Read the model definition and answer for the solid it produces. Units are mm, in the model's axes. Coordinates: 2 decimals unless noted, no trailing zeros. Order: outer loops, then holes, each group sorted by start corner. A loop starts at its lowest first (then second) coordinate and runs counter-clockwise, first axis right, second up. Notation, with made-up numbers: (69, -31.5) -> (102, -31.5) arc R28 ccw to (102, -11.5) -> close; hole circle Ø6 at (-30, 26.5). An arc over 180 degrees is marked (long way). Return JSON: item names as keys, results as strings. Group by question number.
```python
from build123d import *

# Parameters (mm, degrees)
SKETCH1_R           = 2
BOSS_EXTRUDE1_DEPTH = 32.766
SKETCH2_W           = 0.5
SKETCH2_H           = 0.2
SKETCH3_W           = 0.15
SKETCH3_H           = 0.2
CUT_EXTRUDE1_DEPTH  = 3


with BuildPart() as part:
    # Sketch1 → Boss-Extrude1 (new body)
    with BuildSketch(Plane(origin=(0, 0, 0), x_dir=(1, 0, 0), z_dir=(0, 1, 0))):
        Circle(SKETCH1_R)
    extrude(amount=BOSS_EXTRUDE1_DEPTH)

    # Sketch2 → Cut-Revolve1 (revolve, cut)
    with BuildSketch(Plane(origin=(0, 0, 0), x_dir=(0, 0, -1), z_dir=(1, 0, 0))):
        with Locations((1.75, 0.9)):
            Rectangle(SKETCH2_W, SKETCH2_H)
    revolve(axis=Axis((0, 0, 0), (0, 1, 0)), mode=Mode.SUBTRACT)

    # Sketch3 → Cut-Extrude1 (cut)
    with BuildSketch(Plane(origin=(0, 32.766, 0), x_dir=(1, 0, 0), z_dir=(0, 1, 0))):
        with Locations((-1.925, 0)):
            Rectangle(SKETCH3_W, SKETCH3_H)
    extrude(amount=-CUT_EXTRUDE1_DEPTH, mode=Mode.SUBTRACT)


solid = part.part
```
1. Find section C-C on y = 17.5. Determine the outline of the cut face in (x, z), and give its area (3 significant figures).
2. Straight lines are drawn through the part: L1, parallel to Y at x = 1.4, z = 0.85; L2, parallel to X at y = 30.5, z = 0.05; L3, parallel to Z at x = -0.65, y = 20.5. For each, find the intervals that lie inside material, in ascending order.
3. Find section A-A on x = 0.8. Determine the outline of the cut face in (y, z).
4. Find section B-B on z = -1.15. Determine the outline of the cut face in (x, y), and give its area (3 significant figures).
Result:
{
 "1": {"outline": "circle Ø4 at (0, 0)", "area": "12.6 mm^2"},
 "2": {"L1": "0 to 0.8, 1 to 32.77", "L2": "-1.85 to 2", "L3": "-1.89 to 1.89"},
 "3": {"outline": "(0, -1.83) -> (0.8, -1.83) -> (0.8, -1.27) -> (1, -1.27) -> (1, -1.83) -> (32.77, -1.83) -> (32.77, 1.83) -> (1, 1.83) -> (1, 1.27) -> (0.8, 1.27) -> (0.8, 1.83) -> (0, 1.83) -> close"},
 "4": {"outline": "(-1.64, 0) -> (1.64, 0) -> (1.64, 0.8) -> (0.96, 0.8) -> (0.96, 1) -> (1.64, 1) -> (1.64, 32.77) -> (-1.64, 32.77) -> (-1.64, 1) -> (-0.96, 1) -> (-0.96, 0.8) -> (-1.64, 0.8) -> close", "area": "107 mm^2"}
}
